```python
from build123d import *

# Parameters (mm, degrees)
SKETCH_1_W          = 233.345237792
SKETCH_1_H          = 110
SKETCH_1_R          = 1.5
EXTRUDE_1_DEPTH     = 1
SKETCH_2_W          = 70
SKETCH_2_H          = 30
CUT_EXTRUDE_1_DEPTH = 258.974804971
SKETCH_3_R          = 1.5
CUT_EXTRUDE_2_DEPTH = 258.974804971
SKETCH_4_R          = 90
CUT_EXTRUDE_3_DEPTH = 258.974804971


with BuildPart() as part:
    # 草图1 → 凸台-拉伸1 (new body)
    with BuildSketch(Plane.XY):
        with Locations((116.672618896, 55)):
            Rectangle(SKETCH_1_W, SKETCH_1_H)
        with Locations((10, 107)):
            Circle(SKETCH_1_R, mode=Mode.SUBTRACT)
        with Locations((30, 107)):
            Circle(SKETCH_1_R, mode=Mode.SUBTRACT)
        with Locations(Location((203.345237792, 107, 0), (0, 0, 180))):
            Circle(SKETCH_1_R, mode=Mode.SUBTRACT)
        with Locations(Location((223.345237792, 107, 0), (0, 0, 180))):
            Circle(SKETCH_1_R, mode=Mode.SUBTRACT)
    extrude(amount=EXTRUDE_1_DEPTH)

    # 草图2 → 切除-拉伸1 (cut, through all)
    with BuildSketch(Plane.XY.offset(1)):
        with Locations((198.345237792, 95)):
            Rectangle(SKETCH_2_W, SKETCH_2_H)
    extrude(amount=-CUT_EXTRUDE_1_DEPTH, mode=Mode.SUBTRACT)

    # 草图3 → 切除-拉伸2 (cut, through all)
    with BuildSketch(Plane.XY.offset(1)):
        with Locations((10, 107)):
            Circle(SKETCH_3_R)
        with Locations((30, 107)):
            Circle(SKETCH_3_R)
        with Locations(Location((133.345237792, 107, 0), (0, 0, 180))):
            Circle(SKETCH_3_R)
        with Locations(Location((153.345237792, 107, 0), (0, 0, 180))):
            Circle(SKETCH_3_R)
    extrude(amount=-CUT_EXTRUDE_2_DEPTH, mode=Mode.SUBTRACT)

    # 草图4 → 切除-拉伸3 (cut, through all)
    with BuildSketch(Plane.XY.offset(1)):
        with Locations((116.672618896, -30)):
            Circle(SKETCH_4_R)
    extrude(amount=-CUT_EXTRUDE_3_DEPTH, mode=Mode.SUBTRACT)


solid = part.part
```
Part model, mm, in its own coordinate system. Round coordinates to 2 decimals unless told otherwise and drop trailing zeros. Loops run counter-clockwise (first coordinate to the right, second up) from the corner with the lowest first, then second, coordinate; pieces in that order, holes last.
Item 1: Drill centre lines: line 1 (X direction, y = 107, z = 0.6); line 2 (Y direction, x = 10, z = 0.5); line 3 (X direction, y = 20, z = 0.2). Where is each one in solid material? Low to high.
Item 2: Cut at B-B, the plane z = 0.55. Give the cut face in (x, y).
Item 3: Mould opens along X. For faces 1 (the face through (118.224, 59.987, 0.507)), 2 (the face through (89, 68, 1)) say: +X half, -X half, draft (parallel to the pull), parting line (faces both ways), or undercut.
Item 4: Cut at D-D, the plane x = 74. Give the cut face in (y, z), then the cut area to 3 significant figures.
Item 5: Cut at C-C, the plane y = 83. Give the cut face in (x, z).
Item 6: Cut at A-A, the plane y = 22. Give the cut face in (x, z).
A:
1. line 1: x = 0 to 8.5, 11.5 to 28.5, 31.5 to 131.85, 134.85 to 151.85, 154.85 to 163.35
1. line 2: y = 0 to 105.5, 108.5 to 110
1. line 3: x = 0 to 41.84, 191.51 to 233.35
2. outline: (0, 0) - (31.82, 0) arc R90 cw to (201.53, 0) - (233.35, 0) - (233.35, 80) - (163.35, 80) - (163.35, 110) - (0, 110) - close; hole circle Ø3 at (10, 107); hole circle Ø3 at (30, 107); hole circle Ø3 at (133.35, 107); hole circle Ø3 at (153.35, 107)
3. face 1: undercut
3. face 2: draft
4. outline: (49.24, 0) - (110, 0) - (110, 1) - (49.24, 1) - close
4. area: 60.8 mm2
5. outline: (0, 0) - (163.35, 0) - (163.35, 1) - (0, 1) - close
6. outline: (0, 0) - (43.22, 0) - (43.22, 1) - (0, 1) - close; (190.13, 0) - (233.35, 0) - (233.35, 1) - (190.13, 1) - close
